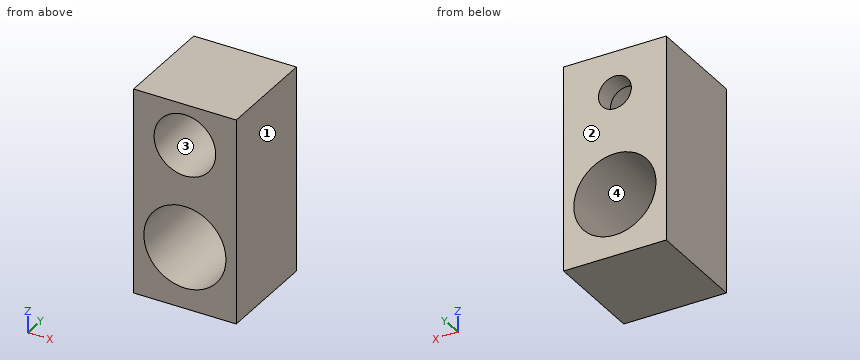
from build123d import *

# Parameters (mm, degrees)
SKETCH1_W           = 10
SKETCH1_H           = 20
SKETCH1_R           = 4
SKETCH1_R_2         = 1.6
BOSS_EXTRUDE1_DEPTH = 10
SKETCH2_R           = 3
CUT_EXTRUDE1_DEPTH  = 8


with BuildPart() as part:
    # Sketch1 → Boss-Extrude1 (new body)
    with BuildSketch(Plane(origin=(0, 0, 0), x_dir=(1, 0, 0), z_dir=(0, 1, 0))):
        with Locations((5, -10)):
            Rectangle(SKETCH1_W, SKETCH1_H)
        with Locations((5, -6)):
            Circle(SKETCH1_R, mode=Mode.SUBTRACT)
        with Locations((5, -16)):
            Circle(SKETCH1_R_2, mode=Mode.SUBTRACT)
    extrude(amount=BOSS_EXTRUDE1_DEPTH)

    # Sketch2 → Cut-Extrude1 (cut)
    with BuildSketch(Plane.XZ):
        with Locations((5, 16)):
            Circle(SKETCH2_R)
    extrude(amount=-CUT_EXTRUDE1_DEPTH, mode=Mode.SUBTRACT)


solid = part.part
The model under review builds one solid part; all positions refer to its coordinate system, in mm. Face numbers are marked on the shaded views. Round coordinates to 2 decimals unless told otherwise and drop trailing zeros. Order: outer loops, then holes, each group sorted by start corner. A loop starts at its lowest first (then second) coordinate and runs counter-clockwise, first axis right, second up. Notation, with made-up numbers: (66.5, 78.5) -> (113.5, 78.5) arc R31 cw to (113.5, 108.5) -> close; hole circle Ø1 at (7, 79). An arc over 180 degrees is marked (long way). Use CSV: the item, a comma, the result in double quotes. Start each with the question number.
(1) Consider section D-D on y = 8.25. Write out the cut boundary in (x, z).
(2) Consider section B-B on x = 5. Write out the cut boundary in (y, z), and give its area (3 significant figures).
(3) Consider section A-A on z = 6. Write out the cut boundary in (x, y).
(4) Insertion check: pin 1 (1.5 mm diameter, centred on y = 7.5, z = 13, fed in from -X). The pin has a flat end and moves straight along its axis. Give the tip position at first contact, or say it passes through.
(5) Wall thickness on probe 1 along Z at (x, y) = (5, 5.75); probe 2 along Z at (x, y) = (5.75, 4); probe 3 along X at (y, z) = (9.5, 16): over which ranges is each line inside the solid? List them lowest first. Write a range as from..to.
(6) Mouldability with a two-part tool opening along X and no side actions: class the marked faces 1, 2, 3 and 4 as pulls with the +X half, pulls with the -X half, needs draft (parallel to the pull), parting line crosses it, or undercut.
(7) Consider section C-C on x = 7.75. Write out the cut boundary in (y, z), and give its area (3 significant figures).
Responses:
1,outline,"(0, 0) -> (10, 0) -> (10, 20) -> (0, 20) -> close; hole circle Ø8 at (5, 6); hole circle Ø3.2 at (5, 16)"
2,outline,"(0, 0) -> (10, 0) -> (10, 2) -> (0, 2) -> close; (0, 10) -> (10, 10) -> (10, 14.4) -> (8, 14.4) -> (8, 13) -> (0, 13) -> close; (0, 19) -> (8, 19) -> (8, 17.6) -> (10, 17.6) -> (10, 20) -> (0, 20) -> close"
2,area,"65.6 mm²"
3,outline,"(0, 0) -> (1, 0) -> (1, 10) -> (0, 10) -> close; (9, 0) -> (10, 0) -> (10, 10) -> (9, 10) -> close"
4,pin 1,"x = 0"
5,probe 1,"0..2, 10..13, 19..20"
5,probe 2,"0..2.07, 9.93..13.1, 18.9..20"
5,probe 3,"0..3.4, 6.6..10"
6,face 1,"pulls with the +X half"
6,face 2,"needs draft"
6,face 3,"undercut"
6,face 4,"undercut"
7,outline,"(0, 0) -> (10, 0) -> (10, 3.1) -> (0, 3.1) -> close; (0, 8.9) -> (10, 8.9) -> (10, 20) -> (0, 20) -> (0, 17.2) -> (8, 17.2) -> (8, 14.8) -> (0, 14.8) -> close"
7,area,"123 mm²"
